Design review of the part shown in the three views and the two pictorial views. Dimensions are in mm from the part's minimum x, y and z. A direction names the side the tool comes from. Round coordinates to 2 decimals unless told otherwise and drop trailing zeros. Loops run counter-clockwise (first coordinate to the right, second up) from the corner with the lowest first, then second, coordinate; pieces in that order, holes last. Notation, with made-up numbers: M 89,-30.75 L 115,-30.75 A19 ccw 115,-3.75 Z; hole C 59,52.5 d5. An arc over 180 degrees is marked long. One line per question, with ' | ' between items. Start each with the question number.
1) For the marked faces 1 and 2, list the 3-axis set-ups (+Z, -Z, +X, -X, +Y, -Y) from which the entire face can be reached by the end or side of a thin tool; tool diameter is ignored.
2) For pin 1 Ø5 at (y, z) = (24.5, 3.5) entering from -X; pin 2 Ø3 at (x, z) = (180, 3) entering from -Y; pin 3 Ø6 at (x, y) = (196.5, 111) entering from +Z; pin 4 Ø1.5 at (x, y) = (139.5, 87) entering from -Z, all flat-tipped, find the tip position at first contact; note any pin that passes through.
3) For probe 1 along Y at (x, z) = (332, 3); probe 2 along Z at (x, y) = (294, 58.5), list the stretches that pass through material, from the lowest coordinate up. Write a range as from..to.
4) We need section B-B (y = 129). Give the boundary of the cut face in (x, z).
5) We need section A-A (x = 181). Give the boundary of the cut face in (y, z).
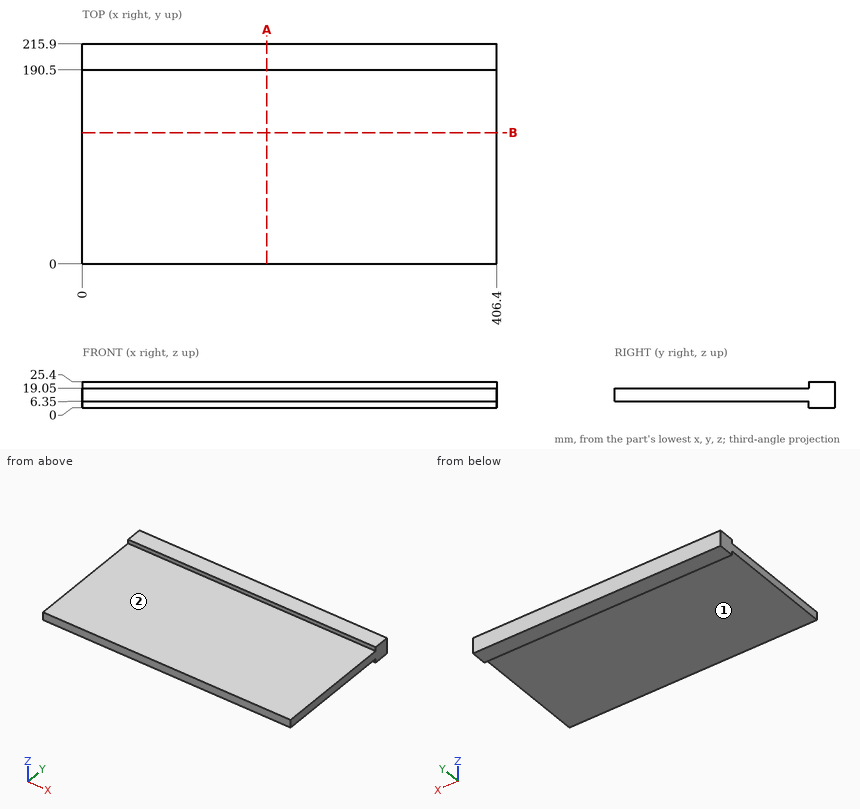
Answers below:
1) face 1: -Z, +X, -X, -Y | face 2: +Z, +X, -X, -Y
2) pin 1: through | pin 2: y = 190.5 | pin 3: z = 19.05 | pin 4: z = 6.35
3) probe 1: 190.5..215.9 | probe 2: 6.35..19.05
4) outline: M 0,6.35 L 406.4,6.35 L 406.4,19.05 L 0,19.05 Z
5) outline: M 0,6.35 L 190.5,6.35 L 190.5,0 L 215.9,0 L 215.9,25.4 L 190.5,25.4 L 190.5,19.05 L 0,19.05 Z
